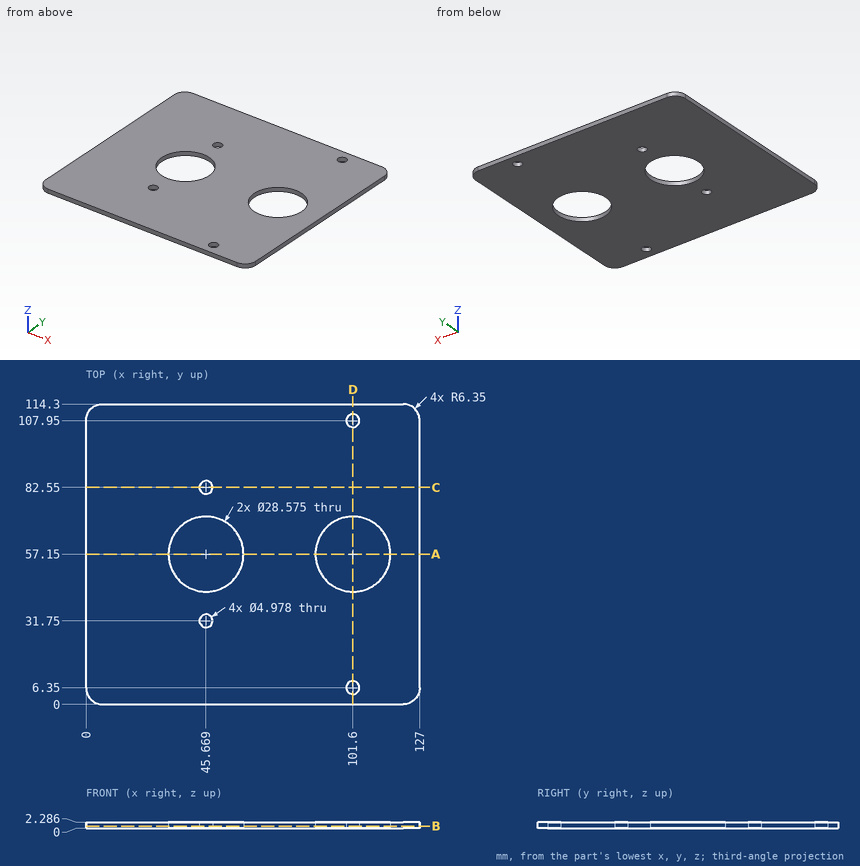
Verification items for this drawing (mm, ordinates from the low corner). Round coordinates to 2 decimals unless told otherwise and drop trailing zeros. Order: outer loops, then holes, each group sorted by start corner. A loop starts at its lowest first (then second) coordinate and runs counter-clockwise, first axis right, second up. Notation, with made-up numbers: M -17,78 L 42,78 A19 ccw 42,87 Z; hole C -13,2 d11. An arc over 180 degrees is marked long. Answer in a Markdown table with one row per item. Add a question column.
Item 1: Sectioned sample at A-A, the plane y = 57.15. Enter the section's corners in (x, z).
Item 2: Sectioned sample at C-C, the plane y = 82.55. Enter the section's corners in (x, z), plus the area to 3 significant figures.
Item 3: Depth check by flat-ended pin: pin 1 Ø23 at (x, y) = (45.67, 57.15) entering from +Z (1 decimal). Enter the tip coordinate at first touch or a pass-through.
Item 4: Material ranges on L1, parallel to Y at x = 101.6, z = 0.75; L2, parallel to Y at x = 44.5, z = 1.7; L3, parallel to X at y = 63, z = 0.7 (1 decimal), recorded low to high. Write a range as [from, to].
Item 5: Sectioned sample at B-B, the plane z = 0.85. State how many separate pieces and enclosed holes the cut face has, plus the area to 3 significant figures.
Item 6: Sectioned sample at D-D, the plane x = 101.6. Enter the section's corners in (y, z).
Filled in:
| question | item | result |
|---|---|---|
| 1 | outline | M 0,0 L 31.38,0 L 31.38,2.29 L 0,2.29 Z; M 59.96,0 L 87.31,0 L 87.31,2.29 L 59.96,2.29 Z; M 115.89,0 L 127,0 L 127,2.29 L 115.89,2.29 Z |
| 2 | outline | M 0,0 L 43.18,0 L 43.18,2.29 L 0,2.29 Z; M 48.16,0 L 127,0 L 127,2.29 L 48.16,2.29 Z |
| 2 | area | 279 mm² |
| 3 | pin 1 | passes through |
| 4 | L1 | y = [0, 3.86], [8.84, 42.86], [71.44, 105.46], [110.44, 114.3] |
| 4 | L2 | y = [0, 29.55], [33.95, 42.91], [71.39, 80.35], [84.75, 114.3] |
| 4 | L3 | x = [0, 32.6], [58.7, 88.6], [114.6, 127] |
| 5 | separate pieces | 1 |
| 5 | enclosed holes | 6 |
| 5 | area | 13,100 mm² |
| 6 | outline | M 0,0 L 3.86,0 L 3.86,2.29 L 0,2.29 Z; M 8.84,0 L 42.86,0 L 42.86,2.29 L 8.84,2.29 Z; M 71.44,0 L 105.46,0 L 105.46,2.29 L 71.44,2.29 Z; M 110.44,0 L 114.3,0 L 114.3,2.29 L 110.44,2.29 Z |
